from build123d import *

# Parameters (mm, degrees)
SKETCH1_R                = 1.55
SKETCH1_R_2              = 1.5
SKETCH1_R_3              = 4.5
SKETCH1_R_4              = 4
SKETCH1_W                = 4
SKETCH1_H                = 5
BOSS_EXTRUDE1_DEPTH      = 4
OTW_R_3_0_3_1_AT_2_COUNT = 2
OTW_R_3_0_3_1_AT_2_PITCH = 17.5


with BuildPart() as part:
    # Sketch1 → Boss-Extrude1 (new body)
    with BuildSketch(Plane(origin=(0, 0, 0), x_dir=(1, 0, 0), z_dir=(0, 1, 0))):
        with BuildLine():
            Line((45, -11.5), (45, 11.5))
            Line((45, 11.5), (65, 11.5))
            Line((65, 11.5), (65, 33))
            ThreePointArc((65, 33), (62.949747468, 37.949747468), (58, 40))
            Line((58, 40), (-58, 40))
            ThreePointArc((-58, 40), (-62.949747468, 37.949747468), (-65, 33))
            Line((-65, 33), (-65, 11.5))
            Line((-65, 11.5), (-45, 11.5))
            Line((-45, 11.5), (-45, -11.5))
            Line((-45, -11.5), (-65, -11.5))
            Line((-65, -11.5), (-65, -33))
            ThreePointArc((-65, -33), (-62.949747468, -37.949747468), (-58, -40))
            Line((-58, -40), (58, -40))
            ThreePointArc((58, -40), (62.949747468, -37.949747468), (65, -33))
            Line((65, -33), (65, -11.5))
            Line((65, -11.5), (45, -11.5))
        make_face()
        with Locations(Location((58, 33, 0), (0, 0, 270))):
            Circle(SKETCH1_R, mode=Mode.SUBTRACT)
        with Locations(Location((58, -33, 0), (0, 0, 270))):
            Circle(SKETCH1_R, mode=Mode.SUBTRACT)
        with Locations(Location((-58, -33, 0), (0, 0, 270))):
            Circle(SKETCH1_R, mode=Mode.SUBTRACT)
        with Locations(Location((-58, 33, 0), (0, 0, 270))):
            Circle(SKETCH1_R, mode=Mode.SUBTRACT)
        with Locations(Location((33.5, 34, 0), (0, 0, 270))):
            Circle(SKETCH1_R_2, mode=Mode.SUBTRACT)
        with Locations(Location((-33.5, 34, 0), (0, 0, 90))):
            Circle(SKETCH1_R_2, mode=Mode.SUBTRACT)
        with Locations(Location((-40.847291444, -35.157580257, 0), (0, 0, 270))):
            Circle(SKETCH1_R_2, mode=Mode.SUBTRACT)
        with Locations(Location((0, -35.15624759, 0), (0, 0, 270))):
            Circle(SKETCH1_R, mode=Mode.SUBTRACT)
        with Locations(Location((40.847291444, -35.157580257, 0), (0, 0, 90))):
            Circle(SKETCH1_R_2, mode=Mode.SUBTRACT)
        with Locations(Location((0, -10, 0), (0, 0, 270))):
            Circle(SKETCH1_R_3, mode=Mode.SUBTRACT)
        with Locations(Location((0, 10, 0), (0, 0, 90))):
            Circle(SKETCH1_R_3, mode=Mode.SUBTRACT)
        with Locations(Location((21.434820624, -23, 0), (0, 0, 270))):
            Circle(SKETCH1_R_4, mode=Mode.SUBTRACT)
        with Locations(Location((-21.434820624, -23, 0), (0, 0, 90))):
            Circle(SKETCH1_R_4, mode=Mode.SUBTRACT)
        with Locations(Location((-21.434820624, 23, 0), (0, 0, 270))):
            Circle(SKETCH1_R_4, mode=Mode.SUBTRACT)
        with Locations(Location((21.434820624, 23, 0), (0, 0, 90))):
            Circle(SKETCH1_R_4, mode=Mode.SUBTRACT)
        with Locations((53, -25.5)):
            Rectangle(SKETCH1_W, SKETCH1_H, mode=Mode.SUBTRACT)
        with Locations((53, 25.5)):
            Rectangle(SKETCH1_W, SKETCH1_H, mode=Mode.SUBTRACT)
        with Locations((-53, -25.5)):
            Rectangle(SKETCH1_W, SKETCH1_H, mode=Mode.SUBTRACT)
        with Locations((-53, 25.5)):
            Rectangle(SKETCH1_W, SKETCH1_H, mode=Mode.SUBTRACT)
    extrude(amount=BOSS_EXTRUDE1_DEPTH)

    # Szkic5 → Otwór Ø3.0 (3)1 (revolve, cut)
    with BuildSketch(Plane(origin=(-45, 2, -8.75), x_dir=(0, 0, 1), z_dir=(0, 1, 0))):
        Polygon((0, 0), (0, 20.901290929), (1.5, 20), (1.5, 0.025), (1.525, 0), align=None)
    otw_r_3_0_3_1 = revolve(axis=Axis((-51.35, 2, -8.75), (1, 0, 0)), mode=Mode.SUBTRACT)

    # Otwór Ø3.0 (3)1 at 2: Otwór Ø3.0 (3)1 ×2
    with Locations(*[(0, 0, i * OTW_R_3_0_3_1_AT_2_PITCH) for i in range(1, OTW_R_3_0_3_1_AT_2_COUNT)]):
        add(otw_r_3_0_3_1, mode=Mode.SUBTRACT)

    # Lustro1: Otwór Ø3.0 (3)1 across plane
    add(otw_r_3_0_3_1.mirror(Plane(origin=(0, 0, 0), x_dir=(0, 0, 1), z_dir=(1, 0, 0))), mode=Mode.SUBTRACT)

    # Lustro1 copy 1 sketch → Lustro1 copy 1 (revolve, cut)
    with BuildSketch(Plane(origin=(45, 2, 8.75), x_dir=(0, 0, 1), z_dir=(0, 1, 0))):
        Polygon((0, 0), (0, -20.901290929), (1.5, -20), (1.5, -0.025), (1.525, 0), align=None)
    revolve(axis=Axis((51.35, 2, 8.75), (1, 0, 0)), mode=Mode.SUBTRACT)


solid = part.part
Build history of the part. All positions in model axes, mm. A direction names the side the tool comes from. Coordinates: 2 decimals unless noted, no trailing zeros. Order: outer loops, then holes, each group sorted by start corner. A loop starts at its lowest first (then second) coordinate and runs counter-clockwise, first axis right, second up. Notation, with made-up numbers: (80, -24) - (127, -24) arc R28 ccw to (127, 12) - close; hole circle Ø9 at (62, 43). An arc over 180 degrees is marked (long way). Put each result on its own line as item: value.
1. Probe line 1 along X through (y, z) = (2.45, 33); line 2 along Z through (x, y) = (29, 1.8); line 3 along Z through (x, y) = (53.5, 0.45). List the from-to ranges inside material, lowest first. Write a range as [from, to].
Answer sheet:
line 1: x = [-65, -59.55], [-56.45, 56.45], [59.55, 65]
line 2: z = [-40, -10.24], [-7.26, 7.26], [10.24, 40]
line 3: z = [-40, -28], [-23, -11.5], [11.5, 23], [28, 40]
2. Saw through at A-A (x = 33.5). Write the cut outline in (y, z).
Answer sheet:
outline: (0, -40) - (4, -40) - (4, -35.5) - (0, -35.5) - close; (0, -32.5) - (4, -32.5) - (4, 40) - (0, 40) - close; hole circle Ø3 at (2, -8.75); hole circle Ø3 at (2, 8.75)
3. Saw through at B-B (x = 0). Write the cut outline in (y, z), and give its area (3 significant figures).
Answer sheet:
outline: (0, -40) - (4, -40) - (4, -14.5) - (0, -14.5) - close; (0, -5.5) - (4, -5.5) - (4, 5.5) - (0, 5.5) - close; (0, 14.5) - (4, 14.5) - (4, 33.61) - (0, 33.61) - close; (0, 36.71) - (4, 36.71) - (4, 40) - (0, 40) - close
area: 236 mm^2
4. Pull direction Z, two halves, no side cores. Call faces 3 (the face through (62.9, 2, 38)), 4 (the face through (65, 2, -22)), 5 (the face through (18.731, 1.972, -20.052)): pulls with the +Z half, pulls with the -Z half, needs draft (parallel to the pull), parting line crosses it, or undercut.
Answer sheet:
face 3: pulls with the +Z half
face 4: needs draft
face 5: undercut
5. Saw through at D-D (y = 1.3). Give the number of separate pieces and of enclosed holes in the cut face, and give its area (3 significant figures).
Answer sheet:
separate pieces: 1
enclosed holes: 19
area: 8,750 mm^2
6. Saw through at C-C (z = 2). Write the cut outline in (x, y), and give its area (3 significant figures).
Answer sheet:
outline: (-45, 0) - (45, 0) - (45, 4) - (-45, 4) - close
area: 360 mm^2
7. Tool access for faces 1 (the face through (-51, 2, 26)), 2 (the face through (-63, 2, 37.9)): list every direction of +Z, -Z, +X, -X, +Y, -Y with a clear straight run to the whole face (end or side of a thin tool).
Answer sheet:
face 1: +Y, -Y
face 2: +Z, -X, +Y, -Y
8. Drop a flat-ended pin along its axis: P1, Ø1, axis at y = 3, z = 10.5, coming from the +X side. Give the stop position or say it passes through.
Answer sheet:
P1: stops at x = 45
